Verification items for this drawing (mm, ordinates from the low corner). Coordinates: 2 decimals unless noted, no trailing zeros. Write each loop counter-clockwise with the first axis right and the second up, starting at its lowest first coordinate (ties: lowest second). Pieces come first, ordered by that corner, then holes. Notation, with made-up numbers: M 46.25,52.25 L 103.25,52.25 A15 ccw 103.25,80.25 Z; hole C 89.5,-3 d8. An arc over 180 degrees is marked long. Write each question's results on one line, items separated by ' | '.
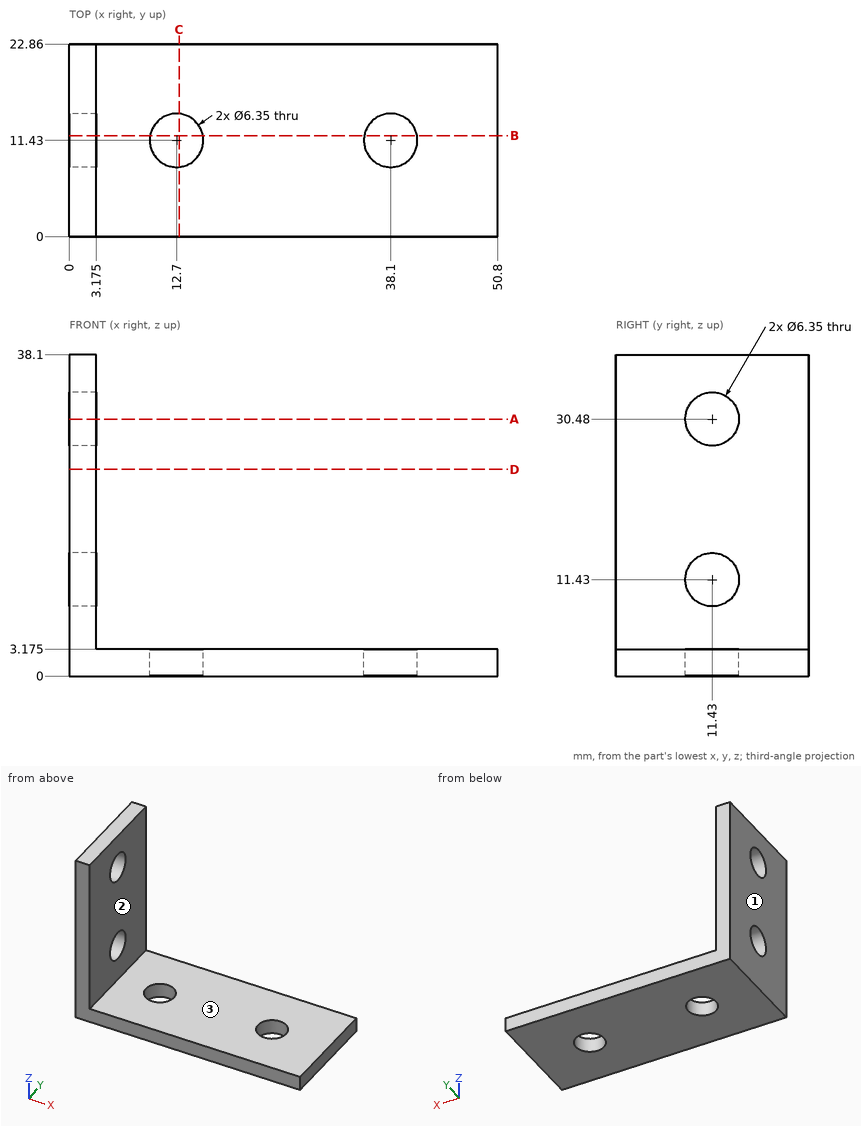
Q1. Sectioned sample at A-A on z = 30.48. Record the cut outline in (x, y) (3 decimals).
Geometry check:
outline: M 0,0 L 3.175,0 L 3.175,8.255 L 0,8.255 Z; M 0,14.605 L 3.175,14.605 L 3.175,22.86 L 0,22.86 Z
Q2. Depth check by flat-ended pin: P1, Ø5, axis at y = 8, z = 19, coming from the +X side (3 decimals); P2, Ø1, axis at x = 34.5, y = 18.5, coming from the +Z side (3 decimals). Enter the tip coordinate at first touch or a pass-through.
Geometry check:
P1: stops at x = 3.175 | P2: stops at z = 3.175
Q3. Mould release check, pull along X, two halves, no side actions. Record for the marked faces 1, 2 and 3: pulls with the +X half, pulls with the -X half, needs draft (parallel to the pull), parting line crosses it, or undercut.
Geometry check:
face 1: pulls with the -X half | face 2: pulls with the +X half | face 3: needs draft
Q4. Scan lines: probe 1 along Y at (x, z) = (38.1, 2.45) (3 decimals); probe 2 along X at (y, z) = (12.75, 2); probe 3 along Z at (x, y) = (21.5, 8.5) (3 decimals). Record each from-to range of solid material in increasing order.
Geometry check:
probe 1: y = 0 to 8.255, 14.605 to 22.86 | probe 2: x = 0 to 9.81, 15.59 to 35.21, 40.99 to 50.8 | probe 3: z = 0 to 3.175
Q5. Sectioned sample at D-D on z = 24.5. Record the cut outline in (x, y) (3 decimals).
Geometry check:
outline: M 0,0 L 3.175,0 L 3.175,22.86 L 0,22.86 Z
Q6. Sectioned sample at B-B on y = 12. Record the cut outline in (x, z) (3 decimals), and give its area (3 significant figures).
Geometry check:
outline: M 0,0 L 9.577,0 L 9.577,3.175 L 3.175,3.175 L 3.175,8.307 L 0,8.307 Z; M 0,14.553 L 3.175,14.553 L 3.175,27.357 L 0,27.357 Z; M 0,33.603 L 3.175,33.603 L 3.175,38.1 L 0,38.1 Z; M 15.823,0 L 34.977,0 L 34.977,3.175 L 15.823,3.175 Z; M 41.223,0 L 50.8,0 L 50.8,3.175 L 41.223,3.175 Z | area: 193 mm2
Q7. Sectioned sample at C-C on x = 13. Record the cut outline in (y, z) (3 decimals).
Geometry check:
outline: M 0,0 L 8.269,0 L 8.269,3.175 L 0,3.175 Z; M 14.591,0 L 22.86,0 L 22.86,3.175 L 14.591,3.175 Z
